Study the drawing (mm; zero at the part's minimum x, y, z) and answer. A direction names the side the tool comes from. Round coordinates to 2 decimals unless told otherwise and drop trailing zeros. Write each loop counter-clockwise with the first axis right and the second up, starting at its lowest first coordinate (ties: lowest second). Pieces come first, ordered by that corner, then holes. Notation, with made-up numbers: M 2,2 L 57,2 A23 ccw 57,33 Z; hole C -15.75,24.5 d6. An arc over 180 degrees is marked long. Write each question's results on one line, items separated by ' | '.
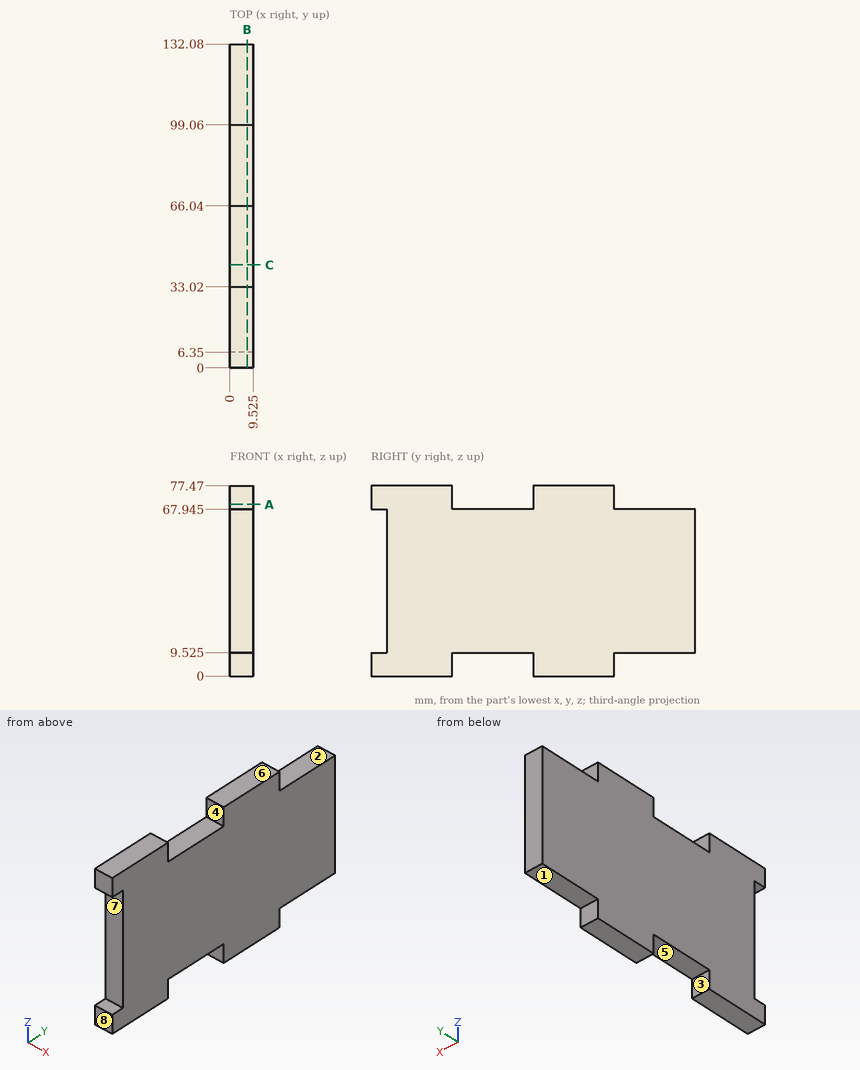
1) The mould has two halves that part along Z. Classify the marked faces 5, 6, 7 and 8: +Z half, -Z half, draft (parallel to the pull), parting line (faces both ways), or undercut.
Return value:
face 5: -Z half | face 6: +Z half | face 7: undercut | face 8: draft
2) Section B-B (x = 7) is taken. Determine the outline of the cut face in (y, z) (3 decimals).
Return value:
outline: M 0,0 L 33.02,0 L 33.02,9.525 L 66.04,9.525 L 66.04,0 L 99.06,0 L 99.06,9.525 L 132.08,9.525 L 132.08,67.945 L 99.06,67.945 L 99.06,77.47 L 66.04,77.47 L 66.04,67.945 L 33.02,67.945 L 33.02,77.47 L 0,77.47 L 0,67.945 L 6.35,67.945 L 6.35,9.525 L 0,9.525 Z
3) Section A-A (z = 70) is taken. Determine the outline of the cut face in (x, y) (3 decimals).
Return value:
outline: M 0,0 L 9.525,0 L 9.525,33.02 L 0,33.02 Z; M 0,66.04 L 9.525,66.04 L 9.525,99.06 L 0,99.06 Z
4) A tool of negligible diameter and unlimited length cuts with its end or side. For the marked faces 1, 2, 3 and 4, from which of +Z, -Z, +X, -X, +Y, -Y can it reach the whole face along a straight path? Write none if from no direction.
Return value:
face 1: -Z, +X, -X, +Y | face 2: +Z, +X, -X, +Y | face 3: -Z, +X, -X | face 4: +Z, +X, -X
5) Section C-C (y = 42) is taken. Determine the outline of the cut face in (x, z) (3 decimals), then the cut area to 3 significant figures.
Return value:
outline: M 0,9.525 L 9.525,9.525 L 9.525,67.945 L 0,67.945 Z | area: 556 mm²
6) Each of these flat-tipped pins is pushed along its axis until it touches: pin 1 (3 mm diameter, centred on x = 4, z = 43.5, fed in from -Y); pin 2 (5 mm diameter, centred on x = 3, y = 56.5, fed in from -Z) (3 decimals); pin 3 (3 mm diameter, centred on x = 6.5, y = 3.5, fed in from -Z); pin 4 (3 mm diameter, centred on x = 7, y = 109, fed in from +Z) (3 decimals). Where does it stop, or does it pass through?
Return value:
pin 1: y = 6.35 | pin 2: z = 9.525 | pin 3: z = 0 | pin 4: z = 67.945
7) Find the intervals of material crossed by line 1 (Y direction, x = 1.5, z = 73.5); line 2 (Z direction, x = 5.75, y = 109) (3 decimals); line 3 (Y direction, x = 4, z = 28), in increasing order.
Return value:
line 1: 0 to 33.02, 66.04 to 99.06 | line 2: 9.525 to 67.945 | line 3: 6.35 to 132.08
